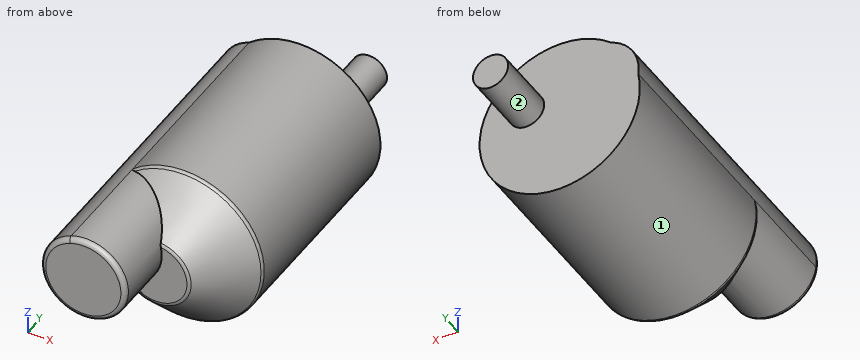
from build123d import *

# Parameters (mm, degrees)
F1_DEPTH    = 500
F0_R        = 27.8691255666
F2_DEPTH    = 400
F3_DEPTH    = 100
F4_SIZE     = 75
F5_R        = 7.62
F6_R        = 7.62
F7_T4_ANGLE = 328.4905382485
F7_S5_R     = 67.3118629199
F7_T6_DEPTH = 190


# Not quite as in the source:
# - a fillet or chamfer that OpenCascade refuses, or shapes differently, is made with other operations: its cross-section is extruded or revolved along the edge and cut away or added


with BuildPart() as f1:
    # F0 (on Front) → F1 (new body)
    with BuildSketch(Plane.XZ):
        with BuildLine():
            ThreePointArc((9.2527889353, 34.7813107073), (-19.6042711183, 90.0272610229), (-81.4330097892, 97.9045711963))
            ThreePointArc((-81.4330097892, 97.9045711963), (-109.241980875, 65.4433324256), (-124.7430483487, 25.6088272504))
            ThreePointArc((-124.7430483487, 25.6088272504), (-53.4620995229, -32.373396615), (9.2527889353, 34.7813107073))
        make_face()
        with BuildLine():
            ThreePointArc((-124.7430483487, 25.6088272504), (-109.241980875, 65.4433324256), (-81.4330097892, 97.9045711963))
            ThreePointArc((-81.4330097892, 97.9045711963), (-115.8022592462, 69.3733827123), (-124.7430483487, 25.6088272504))
        make_face()
    extrude(amount=F1_DEPTH)

    # F0 (on Front) → F2 (join)
    with BuildSketch(Plane.XZ):
        with BuildLine():
            ThreePointArc((-124.7430483487, 25.6088272504), (-12.870314303, -126.6925220927), (127.3445724971, 0))
            ThreePointArc((127.3445724971, 0), (54.0674963619, 115.2967735091), (-81.4330097892, 97.9045711963))
            ThreePointArc((-81.4330097892, 97.9045711963), (-19.6042711183, 90.0272610229), (9.2527889353, 34.7813107073))
            ThreePointArc((9.2527889353, 34.7813107073), (-53.4620995229, -32.373396615), (-124.7430483487, 25.6088272504))
        make_face()
        with Locations((52.5650605559, 30.6920967996)):
            Circle(F0_R, mode=Mode.SUBTRACT)
        with Locations((52.5650605559, 30.6920967996)):
            Circle(F0_R)
    extrude(amount=F2_DEPTH)

    # F0 (on Front) → F3 (join)
    with BuildSketch(Plane.XZ):
        with Locations((52.5650605559, 30.6920967996)):
            Circle(F0_R)
    extrude(amount=-F3_DEPTH)

    # F4
    f4_edges = [f1.edges().sort_by_distance(p)[0] for p in [
        (109.241981, -400, -65.443332),
    ]]
    chamfer(f4_edges, length=F4_SIZE)

    # F5
    f5_edges = [f1.edges().sort_by_distance(p)[0] for p in [
        (-125.370937, -500, 34.781311),
    ]]
    fillet(f5_edges, radius=F5_R)

    # F6
    f6_edges = [f1.edges().sort_by_distance(p)[0] for p in [
        (44.903561, -400, -26.900269),
    ]]
    fillet(f6_edges, radius=F6_R)

    # F7: fillet of radius 7.62 on 1 edges, made by hand


with BuildPart() as f7_tool2:
    # F7_s3 → F7_t4 (revolve)
    with BuildSketch(Plane(origin=(0, 0, 0), x_dir=(0, 1, 0), z_dir=(0.2616792898, 0, 0.9651548836))):
        with BuildLine():
            ThreePointArc((-327.2318463274, 125.1127261697), (-324.7597404093, 126.7645345348), (-321.8436926547, 127.3445724971))
            Line((-321.8436926547, 127.3445724971), (-325, 127.3445724971))
            Line((-325, 127.3445724971), (-327.2318463274, 125.1127261697))
        make_face()
    revolve(axis=Axis((0, -325, 0), (0, -1, 0)), revolution_arc=F7_T4_ANGLE)

    # F7_s5 → F7_t6 (cut, symmetric)
    with BuildSketch(Plane.XZ.offset(321.8)):
        with Locations((-58.0590739846, 34.7813107073)):
            Circle(F7_S5_R)
    extrude(amount=F7_T6_DEPTH, both=True, mode=Mode.SUBTRACT)


with BuildPart() as f1_1:
    add(f1.part)

    # F7_t1: cut F7_tool2
    add(f7_tool2.part, mode=Mode.SUBTRACT)


solid = f1_1.part
Input: part model. Units: mm. Frame: model coordinates. Face numbers are marked on the shaded views. A direction names the side the tool comes from. Round coordinates to 2 decimals unless told otherwise and drop trailing zeros. Loops run counter-clockwise (first coordinate to the right, second up) from the corner with the lowest first, then second, coordinate; pieces in that order, holes last. Notation, with made-up numbers: (12, 16) -> (62, 16) arc R13 ccw to (62, 40) -> close; hole circle Ø10 at (88, 33). An arc over 180 degrees is marked (long way). Answer as a JSON object with one key per item and string values. Group by question number.
1) Section query A-A on y = -423.5. Output: boundary loops of the cut face in (x, z), plus the area to 3 significant figures.
2) Section query C-C on y = -341.5. Output: boundary loops of the cut face in (x, z).
3) Section query B-B on y = -220.5. Output: boundary loops of the cut face in (x, z).
4) Reachability of the marked faces 1 and 2 from +Z, -Z, +X, -X, +Y, -Y: full face, straight path, thin tool, end or side. Return the list, or none.
5) Pin query (flat end, axial travel): pin 1 (4 mm diameter, centred on y = -283.5, z = 87.5, fed in from -X); pin 2 (6 mm diameter, centred on x = -31, y = -271.5, fed in from -Z); pin 3 (10 mm diameter, centred on y = -123, z = 14.5, fed in from +X). Return the tip coordinate at first contact, or that it passes through.
6) Ray query, L1, parallel to Y at x = -18.5, z = 1.5; L2, parallel to Z at x = -5.5, y = -225.5; L3, parallel to Y at x = 101, z = -44.5. Return the intervals inside material, ascending.
Reply:
{
 "1": {"outline": "circle Ø134.62 at (-58.06, 34.78)", "area": "14,200 mm2"},
 "2": {"outline": "(-110.6, -7.29) arc R110.84 ccw (long way) to (-45.76, 100.96) arc R67.31 ccw to start"},
 "3": {"outline": "(-124.74, 25.61) arc R127.34 ccw (long way) to (-81.43, 97.9) arc R67.31 ccw to start"},
 "4": {"face 1": "+Y, -Y", "face 2": "+Y"},
 "5": {"pin 1": "stops at x = -102.31", "pin 2": "stops at z = -124.23", "pin 3": "stops at x = 126.99"},
 "6": {"L1": "y = -500 to 0", "L2": "z = -127.23 to 127.23", "L3": "y = -341.98 to 0"}
}
